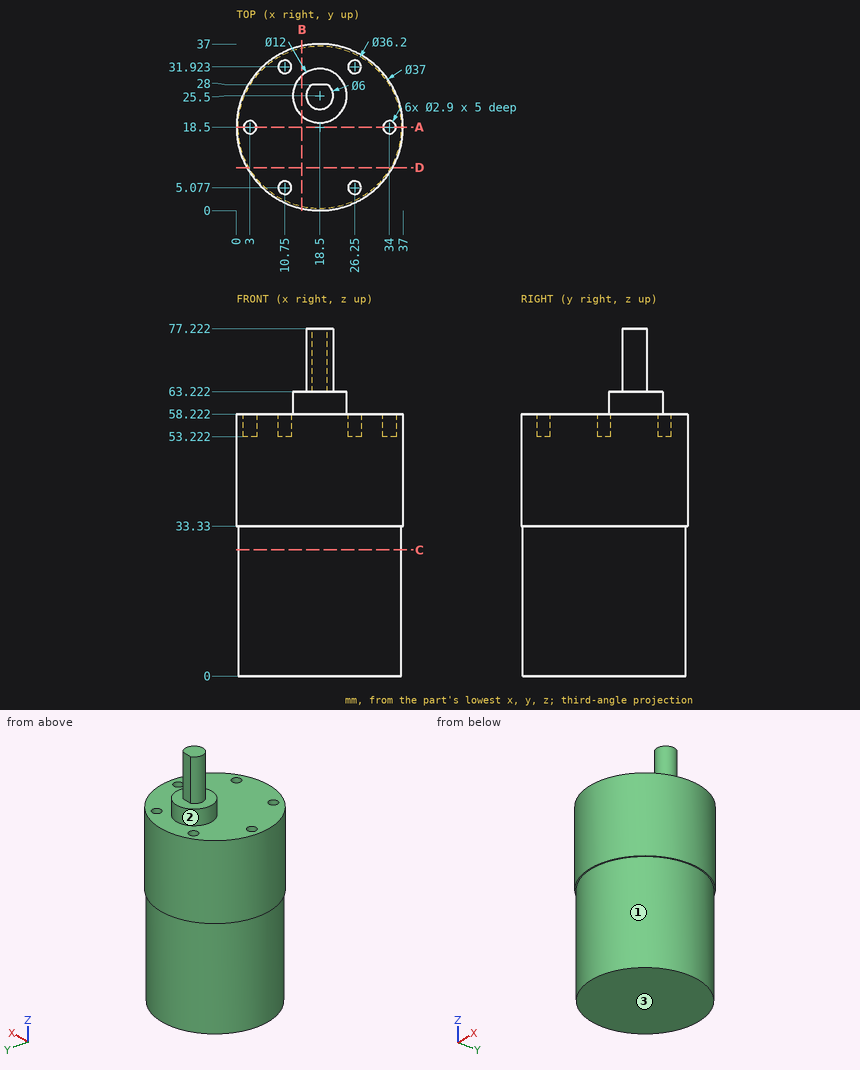
Print and shaded views of the part. All mm, measured from the part's lowest x, y and z. A direction names the side the tool comes from. Give positions to 0.01 mm unless a question says otherwise; leave off trailing zeros. Order: outer loops, then holes, each group sorted by start corner. A loop starts at its lowest first (then second) coordinate and runs counter-clockwise, first axis right, second up. Notation, with made-up numbers: M 80,-24.75 L 127,-24.75 A15 cw 127,-14.75 Z; hole C -17.75,66.5 d8. An arc over 180 degrees is marked long. Use one line per item in the form item = value.
Q1. Slice it at A-A, the plane y = 18.5. Write the cut outline in (x, z), and give its area (3 significant figures).
Conclusion:
outline = M 0,33.33 L 0.4,33.33 L 0.4,0 L 36.6,0 L 36.6,33.33 L 37,33.33 L 37,58.22 L 35.45,58.22 L 35.45,53.22 L 32.55,53.22 L 32.55,58.22 L 4.45,58.22 L 4.45,53.22 L 1.55,53.22 L 1.55,58.22 L 0,58.22 Z
area = 2,100 mm2
Q2. Slice it at B-B, the plane x = 14.5. Write the cut outline in (y, z), and give its area (3 significant figures).
Conclusion:
outline = M 0.44,33.33 L 0.85,33.33 L 0.85,0 L 36.15,0 L 36.15,33.33 L 36.56,33.33 L 36.56,58.22 L 29.97,58.22 L 29.97,63.22 L 21.03,63.22 L 21.03,58.22 L 0.44,58.22 Z
area = 2,120 mm2
Q3. Slice it at D-D, the plane y = 9.5. Write the cut outline in (x, z), and give its area (3 significant figures).
Conclusion:
outline = M 2.34,33.33 L 2.8,33.33 L 2.8,0 L 34.2,0 L 34.2,33.33 L 34.66,33.33 L 34.66,58.22 L 2.34,58.22 Z
area = 1,850 mm2
Q4. Slice it at C-C, the plane z = 28. Write the cut outline in (x, y).
Conclusion:
outline = C 18.5,18.5 d36.2
Q5. Which spindle directions (+Z, -Z, +X, -X, +Y, -Y) get a long thin tool onto all of the face, cutting with end or side? Do the marked faces 1, 2 and 3. Say none if no direction does.
Conclusion:
face_1 = -Z
face_2 = +Z
face_3 = -Z, +X, -X, +Y, -Y
Q6. Wall check: probe 1 along Y at (x, z) = (10.75, 54.7); probe 2 along Z at (x, y) = (31, 8); probe 3 along X at (y, z) = (18, 56). Give the ranges that are in metal, low to high.
Conclusion:
probe_1 = 1.7 to 3.63, 6.53 to 30.47, 33.37 to 35.3
probe_2 = 0 to 58.22
probe_3 = 0.01 to 1.64, 4.36 to 32.64, 35.36 to 36.99
Q7. Pin check, flat tips, straight feed: P1, Ø3, axis at x = 34, y = 18, coming from the +Z side; P2, Ø1.4, axis at x = 26.5, y = 31.5, coming from the +Z side; P3, Ø2, axis at y = 21.5, z = 43.5, coming from the -X side. Stop position of each tip, or through.
Conclusion:
P1 = 58.22
P2 = 53.22
P3 = 0.11
